Design review of the part built by this model. Coordinates are the model's own, in mm. Face numbers are marked on the shaded views. Coordinates: 2 decimals unless noted, no trailing zeros. Loops run counter-clockwise (first coordinate to the right, second up) from the corner with the lowest first, then second, coordinate; pieces in that order, holes last. Notation, with made-up numbers: (37, 84.25) - (89, 84.25) arc R7 ccw to (89, 95.25) - close; hole circle Ø2 at (28, -28.5). An arc over 180 degrees is marked (long way). Answer in a Markdown table with one row per item. Add a question column.
(1) The part is to be moulded in two halves that separate along X. For the marked faces 1, 2, 3 and 4, say which applies: released by +X, released by -X, zero draft, split by the parting line, or undercut.
(2) We need section A-A, the plane z = 22.5. Write out the cut boundary in (x, y).
(3) To check wall thickness, follow L1, parallel to Y at x = 0, z = 10; L2, parallel to Y at x = 0, z = 24; L3, parallel to X at y = -20, z = 21.5. State the ranges of each line that lie inside material, in increasing order. Write a range as [from, to].
(4) We need section B-B, the plane z = 11.5. Write out the cut boundary in (x, y).
(5) Clearance check with flat-ended pins moving along their axes: pin 1 (3 mm diameter, centred on x = 27, z = 16.5, fed in from -Y); pin 2 (11 mm diameter, centred on x = 2.5, y = -3.5, fed in from +Z); pin 3 (3 mm diameter, centred on x = 6, y = 24, fed in from -Z); pin 4 (12 mm diameter, centred on y = 19.5, z = 5, fed in from -X). State where each tip first meets the part, or that it passes through.
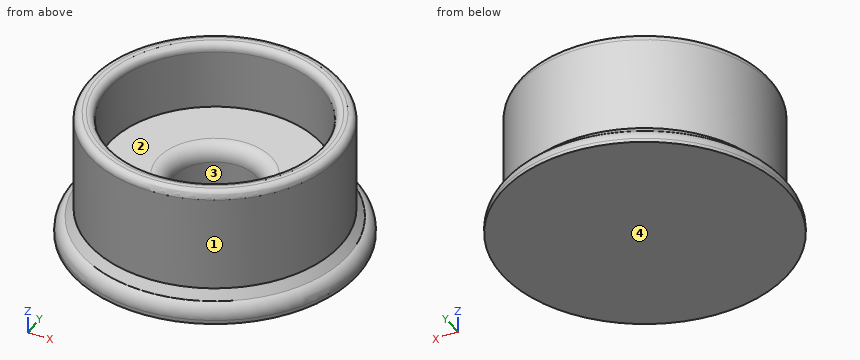
from build123d import *

# Parameters (mm, degrees)
SKETCH_R        = 33
PAD_DEPTH       = 34
SKETCH001_R     = 28
POCKET_DEPTH    = 17.5
SKETCH002_R     = 11
POCKET001_DEPTH = 15.5
SKETCH003_R     = 37.5
SKETCH003_R_2   = 25
PAD001_DEPTH    = 5
FILLET_R        = 4
CHAMFER_SIZE    = 2
FILLET001_R     = 2
FILLET002_R     = 2
FILLET003_R     = 4


with BuildPart() as part:
    # Sketch → Pad (new body)
    with BuildSketch(Plane.XY):
        Circle(SKETCH_R)
    extrude(amount=PAD_DEPTH)

    # Sketch001 (on Face3 of Pad) → Pocket (cut)
    with BuildSketch(Plane.XY.offset(34)):
        Circle(SKETCH001_R)
    extrude(amount=-POCKET_DEPTH, mode=Mode.SUBTRACT)

    # Sketch002 (on Face5 of Pocket) → Pocket001 (cut)
    with BuildSketch(Plane.XY.offset(16.5)):
        Circle(SKETCH002_R)
    extrude(amount=-POCKET001_DEPTH, mode=Mode.SUBTRACT)

    # Sketch003 (on Face2 of Pocket001) → Pad001 (join)
    with BuildSketch(Plane(origin=(0, 0, 0), x_dir=(1, 0, 0), z_dir=(0, 0, -1))):
        Circle(SKETCH003_R)
        Circle(SKETCH003_R_2, mode=Mode.SUBTRACT)
    extrude(amount=-PAD001_DEPTH)

    # Fillet
    fillet_edges = [part.edges().sort_by_distance(p)[0] for p in [
        (-37.5, 0, 5),
    ]]
    fillet(fillet_edges, radius=FILLET_R)

    # Chamfer
    chamfer_edges = [part.edges().sort_by_distance(p)[0] for p in [
        (-33, 0, 5),
    ]]
    chamfer(chamfer_edges, length=CHAMFER_SIZE)

    # Fillet001
    fillet001_edges = [part.edges().sort_by_distance(p)[0] for p in [
        (-33, 0, 34),
    ]]
    fillet(fillet001_edges, radius=FILLET001_R)

    # Fillet002
    fillet002_edges = [part.edges().sort_by_distance(p)[0] for p in [
        (-28, 0, 34),
    ]]
    fillet(fillet002_edges, radius=FILLET002_R)

    # Fillet003
    fillet003_edges = [part.edges().sort_by_distance(p)[0] for p in [
        (-11, 0, 16.5),
    ]]
    fillet(fillet003_edges, radius=FILLET003_R)


solid = part.part
Responses:
| question | item | result |
|---|---|---|
| 1 | face 1 | split by the parting line |
| 1 | face 2 | undercut |
| 1 | face 3 | undercut |
| 1 | face 4 | zero draft |
| 2 | outline | circle Ø66 at (0, 0); hole circle Ø56 at (0, 0) |
| 3 | L1 | y = [-33, -11], [11, 33] |
| 3 | L2 | y = [-33, -28], [28, 33] |
| 3 | L3 | x = [-26.25, -19.6], [19.6, 26.25] |
| 4 | outline | circle Ø66 at (0, 0); hole circle Ø22 at (0, 0) |
| 5 | pin 1 | stops at y = -20.95 |
| 5 | pin 2 | stops at z = 1 |
| 5 | pin 3 | stops at z = 0 |
| 5 | pin 4 | stops at x = -34.53 |
